Work out the finished part from the listing and answer in its coordinate system (mm). Give positions to 0.01 mm unless a question says otherwise; leave off trailing zeros. Order: outer loops, then holes, each group sorted by start corner. A loop starts at its lowest first (then second) coordinate and runs counter-clockwise, first axis right, second up. Notation, with made-up numbers: (27.25, -35.5) - (39.25, -35.5) arc R23 cw to (39.25, -21.5) - close; hole circle Ø9 at (34.25, 2). An arc over 180 degrees is marked (long way). Return JSON: item names as keys, results as strings. Group by question number.
Solid Edge part; units mm, degrees
sketch "Sketch1" plane through (0, 0, 0) normal (0, 0, 1) x (1, 0, 0)
  circle A0 centre (0, 0) radius 145
extrude "Protrusion1" add sketch "Sketch1" along normal blind 11.5
hole "Bohrung_1" at (-20, 0, 11.5) direction (0, 0, -1) diameter 4.917 depth 10 thread major 6 thread length 8
hole "Hole1" at (20, 0, 11.5) direction (0, 0, -1) diameter 4.917 depth 10 thread major 6 thread length 8
hole "Bohrung_3" at (-110, 42.5, 11.5) direction (0, 0, -1) diameter 4.917 depth 10 thread major 6 thread length 8
hole "Hole2" at (-110, 27.5, 11.5) direction (0, 0, -1) diameter 4.917 depth 10 thread major 6 thread length 8
hole "Bohrung_9" at (42.5, -110, 11.5) direction (0, 0, -1) diameter 4.917 depth 10 thread major 6 thread length 8
hole "Hole3" at (27.5, -110, 11.5) direction (0, 0, -1) diameter 4.917 depth 10 thread major 6 thread length 8
1. The part is cut by section C-C (y = 117). Give the vertices of the cut face in (x, z), and give its area (3 significant figures).
2. Each of these flat-tipped pins is pushed along its axis until it touches: pin 1 (4.5 mm diameter, centred on x = -110, y = 27.5, fed in from +Z); pin 2 (3 mm diameter, centred on y = -49, z = 9, fed in from -X); pin 3 (5 mm diameter, centred on y = 66.5, z = 4, fed in from +X). Where does it stop, or does it pass through?
3. The part is cut by section A-A (z = 6). Give the vertices of the cut face in (x, y).
4. The part is cut by section B-B (x = 91). Give the vertices of the cut face in (y, z).
5. Consider probe 1 along Y at (x, z) = (-110, 7.25); probe 2 along Y at (x, z) = (-20, 7.5); probe 3 along Y at (x, z) = (42.5, 3.5). Determine where each line is inside the solid, lowest interval first. Write a range as from..to.
Answers:
{
 "1": {"outline": "(-85.65, 0) - (85.65, 0) - (85.65, 11.5) - (-85.65, 11.5) - close", "area": "1,970 mm^2"},
 "2": {"pin 1": "stops at z = 1.5", "pin 2": "stops at x = -137", "pin 3": "stops at x = 130.11"},
 "3": {"outline": "circle Ø290 at (0, 0); hole circle Ø4.92 at (-110, 27.5); hole circle Ø4.92 at (-110, 42.5); hole circle Ø4.92 at (-20, 0); hole circle Ø4.92 at (20, 0); hole circle Ø4.92 at (27.5, -110); hole circle Ø4.92 at (42.5, -110)"},
 "4": {"outline": "(-112.89, 0) - (112.89, 0) - (112.89, 11.5) - (-112.89, 11.5) - close"},
 "5": {"probe 1": "y = -94.47..25.04, 29.96..40.04, 44.96..94.47", "probe 2": "y = -143.61..-2.46, 2.46..143.61", "probe 3": "y = -138.63..-112.46, -107.54..138.63"}
}
